from build123d import *

# Parameters (mm, degrees)
SKETCH_1_R          = 34
SKETCH_1_R_2        = 30
EXTRUDE_1_DEPTH     = 20
EXTRUDE_START       = 20
SKETCH_1_2_R        = 34
SKETCH_1_2_R_2      = 30
EXTRUDE_2_DEPTH     = 4
SKETCH_2_R          = 11
SKETCH_2_R_2        = 1.5
CUT_EXTRUDE_1_DEPTH = 53.076866265
CHAMFER_1_SIZE      = 2
SKETCH_3_R          = 12.5
SKETCH_3_R_2        = 11
EXTRUDE_3_DEPTH     = 16
EXTRUDE_START_2     = 16
SKETCH_3_2_R        = 12.5
SKETCH_3_2_R_2      = 11
EXTRUDE_4_DEPTH     = 3
SKETCH_5_R          = 2.5
CUT_EXTRUDE_2_DEPTH = 52
EXTRUDE_START_3     = 3
SKETCH_6_R          = 30
SKETCH_6_R_2        = 12.5
EXTRUDE_5_DEPTH     = 3


with BuildPart() as part:
    # 草图1 → 凸台-拉伸1 (new body)
    with BuildSketch(Plane(origin=(0, 0, 0), x_dir=(1, 0, 0), z_dir=(0, 1, 0))):
        with Locations(Location((0, 0, 0), (0, 0, 270))):
            Circle(SKETCH_1_R)
        with Locations(Location((0, 0, 0), (0, 0, 270))):
            Circle(SKETCH_1_R_2, mode=Mode.SUBTRACT)
    extrude(amount=EXTRUDE_1_DEPTH)

    # 草图1<2> → 凸台-拉伸2 (add)
    with BuildSketch(Plane(origin=(0, 0, 0), x_dir=(1, 0, 0), z_dir=(0, 1, 0)).offset(EXTRUDE_START)):
        with Locations(Location((0, 0, 0), (0, 0, 270))):
            Circle(SKETCH_1_2_R)
        with Locations(Location((0, 0, 0), (0, 0, 270))):
            Circle(SKETCH_1_2_R_2, mode=Mode.SUBTRACT)
        with Locations(Location((0, 0, 0), (0, 0, 270))):
            Circle(SKETCH_1_2_R_2)
    extrude(amount=-EXTRUDE_2_DEPTH)

    # 草图2 → 切除-拉伸1 (cut, through all)
    with BuildSketch(Plane(origin=(0, 20, 0), x_dir=(1, 0, 0), z_dir=(0, 1, 0))):
        with Locations(Location((0, 0, 0), (0, 0, 270))):
            Circle(SKETCH_2_R)
        with Locations(Location((0, 15, 0), (0, 0, 270))):
            Circle(SKETCH_2_R_2)
        with Locations(Location((0, 22, 0), (0, 0, 270))):
            Circle(SKETCH_2_R_2)
        with Locations(Location((15, 0, 0), (0, 0, 270))):
            Circle(SKETCH_2_R_2)
        with Locations(Location((22, 0, 0), (0, 0, 270))):
            Circle(SKETCH_2_R_2)
        with Locations(Location((0, -15, 0), (0, 0, 270))):
            Circle(SKETCH_2_R_2)
        with Locations(Location((0, -22, 0), (0, 0, 270))):
            Circle(SKETCH_2_R_2)
        with Locations(Location((-15, 0, 0), (0, 0, 270))):
            Circle(SKETCH_2_R_2)
        with Locations(Location((-22, 0, 0), (0, 0, 270))):
            Circle(SKETCH_2_R_2)
    extrude(amount=-CUT_EXTRUDE_1_DEPTH, mode=Mode.SUBTRACT)

    # 倒角1
    chamfer_1_edges = [part.edges().sort_by_distance(p)[0] for p in [
        (0, 20, -34),
    ]]
    chamfer(chamfer_1_edges, length=CHAMFER_1_SIZE)

    # 草图3 → 凸台-拉伸3 (add)
    with BuildSketch(Plane.XZ.offset(-16)):
        with Locations(Location((0, 0, 0), (0, 0, 90))):
            Circle(SKETCH_3_R)
        with Locations(Location((0, 0, 0), (0, 0, 90))):
            Circle(SKETCH_3_R_2, mode=Mode.SUBTRACT)
    extrude(amount=EXTRUDE_3_DEPTH)

    # 草图3<2> → 凸台-拉伸4 (add)
    with BuildSketch(Plane.XZ.offset(-16).offset(EXTRUDE_START_2)):
        with Locations(Location((0, 0, 0), (0, 0, 90))):
            Circle(SKETCH_3_2_R)
        with Locations(Location((0, 0, 0), (0, 0, 90))):
            Circle(SKETCH_3_2_R_2, mode=Mode.SUBTRACT)
        with Locations(Location((0, 0, 0), (0, 0, 90))):
            Circle(SKETCH_3_2_R_2)
    extrude(amount=-EXTRUDE_4_DEPTH)

    # 草图5 → 切除-拉伸2 (cut, through all)
    with BuildSketch(Plane(origin=(0, 3, 0), x_dir=(1, 0, 0), z_dir=(0, 1, 0))):
        with Locations(Location((0, 0, 0), (0, 0, 270))):
            Circle(SKETCH_5_R)
    extrude(amount=-CUT_EXTRUDE_2_DEPTH, mode=Mode.SUBTRACT)

    # 草图6 → 凸台-拉伸5 (add)
    with BuildSketch(Plane.XZ.offset(-16).offset(EXTRUDE_START_3)):
        with Locations(Location((0, 0, 0), (0, 0, 270))):
            Circle(SKETCH_6_R)
        with Locations(Location((0, 0, 0), (0, 0, 90))):
            Circle(SKETCH_6_R_2, mode=Mode.SUBTRACT)
    extrude(amount=EXTRUDE_5_DEPTH)


solid = part.part
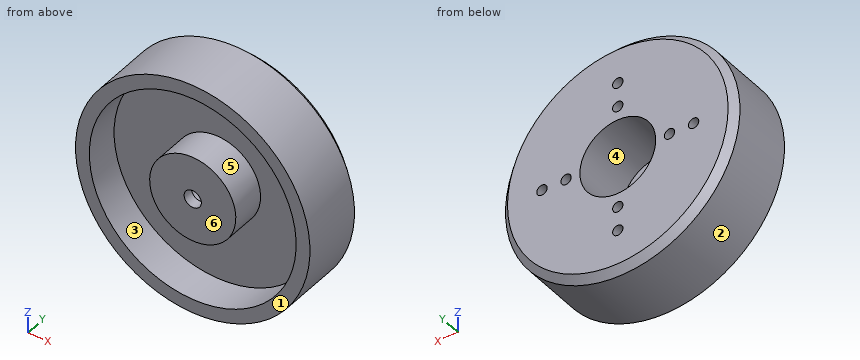
The model under review builds one solid part; all positions refer to its coordinate system, in mm. Face numbers are marked on the shaded views. A direction names the side the tool comes from. Give positions to 0.01 mm unless a question says otherwise; leave off trailing zeros. Order: outer loops, then holes, each group sorted by start corner. A loop starts at its lowest first (then second) coordinate and runs counter-clockwise, first axis right, second up. Notation, with made-up numbers: M 7,36.5 L 54,36.5 A33 ccw 54,71.5 Z; hole C 9.5,-18 d6. An arc over 180 degrees is marked long. Answer in a Markdown table with one row per item. Add a question column.
1. Add section A-A on y = 14. State the section outline as (x, z) points.
2. Add section B-B on z = 0. Count the separate pieces of the cut face and the enclosed holes in it, plus the area to 3 significant figures.
3. To check wall thickness, follow line 1 along X through (y, z) = (1.3, 0); line 2 along X through (y, z) = (7.75, 0); line 3 along X through (y, z) = (17.1, 0). State the ranges of each line that lie inside material, in increasing order.
4. For pin 1 Ø13 at (x, z) = (0, 0) entering from +Y; pin 2 Ø8 at (x, y) = (-4.5, 16.5) entering from -Z; pin 3 Ø8 at (x, y) = (26, 17) entering from -Z, all flat-tipped, find the tip position at first contact; note any pin that passes through.
5. Mouldability with a two-part tool opening along Z and no side actions: class the marked faces 1, 2 and 3 as released by +Z, released by -Z, zero draft, split by the parting line, or undercut.
6. Machinability: for the marked faces 4, 5 and 6, which of the approach directions +Z, -Z, +X, -X, +Y, -Y give a long, thin tool a straight path to every point of the face, cutting with its end or side? Answer none if there is none.
The answers:
| question | item | result |
|---|---|---|
| 1 | outline | C 0,0 d68; C 0,0 d25; hole C 0,0 d60; hole C 0,0 d22 |
| 2 | separate pieces | 4 |
| 2 | enclosed holes | 0 |
| 2 | area | 464 mm2 |
| 3 | line 1 | -34 to -30, -12.5 to -2.5, 2.5 to 12.5, 30 to 34 |
| 3 | line 2 | -34 to -30, -12.5 to -11, 11 to 12.5, 30 to 34 |
| 3 | line 3 | -34 to -23.5, -20.5 to -16.5, -13.5 to -11, 11 to 13.5, 16.5 to 20.5, 23.5 to 34 |
| 4 | pin 1 | y = 3 |
| 4 | pin 2 | z = -34 |
| 4 | pin 3 | z = -25.92 |
| 5 | face 1 | zero draft |
| 5 | face 2 | split by the parting line |
| 5 | face 3 | undercut |
| 6 | face 4 | +Y |
| 6 | face 5 | -Y |
| 6 | face 6 | +Z, -Z, +X, -X, -Y |
